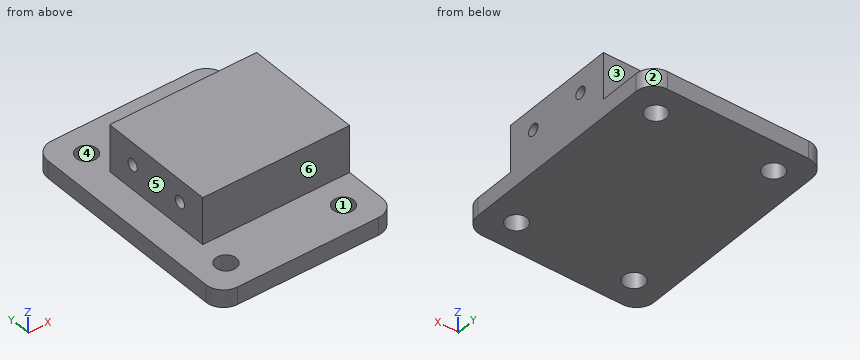
from build123d import *

# Parameters (mm, degrees)
SKETCH_1_W              = 30
SKETCH_1_H              = 40
EXTRUDE_1_DEPTH         = 1.5
SKETCH_2_W              = 25
SKETCH_2_H              = 20
EXTRUDE_2_DEPTH         = 8
HOLE_WIZARD_2_0_2_3_D   = 2
HOLE_WIZARD_3_5_3_5_1_D = 3.5
FILLET_1_R              = 3


with BuildPart() as part:
    # 草圖1 → 填料-伸長1 (new, symmetric)
    with BuildSketch(Plane.XY):
        Rectangle(SKETCH_1_W, SKETCH_1_H)
    extrude(amount=EXTRUDE_1_DEPTH, both=True)

    # 草圖2 → 填料-伸長2 (add)
    with BuildSketch(Plane.XY.offset(1.5)):
        with Locations((2.5, 0)):
            Rectangle(SKETCH_2_W, SKETCH_2_H)
    extrude(amount=EXTRUDE_2_DEPTH)

    # Ø2.0 (2) 直徑孔3 (through all)
    with Locations(Plane.ZY.offset(10)):
        with Locations((5.69, 5.08), (5.69, -5.08)):
            Hole(HOLE_WIZARD_2_0_2_3_D / 2)

    # Ø3.5 (3.5) 直徑孔1 (through all)
    with Locations(Plane.XY.offset(1.5)):
        with Locations((10, 15), (-10, -15), (-10, 15), (10, -15)):
            Hole(HOLE_WIZARD_3_5_3_5_1_D / 2)

    # 圓角1
    fillet_1_edges = [part.edges().sort_by_distance(p)[0] for p in [
        (15, -20, 0),
        (-15, -20, 0),
        (-15, 20, 0),
        (15, 20, 0),
    ]]
    fillet(fillet_1_edges, radius=FILLET_1_R)


solid = part.part
Can you work these out from the model? Positions are in its coordinate system, mm. Face numbers are marked on the shaded views. A direction names the side the tool comes from. Give positions to 0.01 mm unless a question says otherwise; leave off trailing zeros. Loops run counter-clockwise (first coordinate to the right, second up) from the corner with the lowest first, then second, coordinate; pieces in that order, holes last. Notation, with made-up numbers: M -15,31 L 37,31 A21 ccw 37,67 Z; hole C 62.5,78 d8. An arc over 180 degrees is marked long. One line per item, written item: value. Start each with the question number.
1) I'm going to push flat-ended pins straight in: pin 1 (4 mm diameter, centred on x = -3.5, z = 7.5, fed in from -Y); pin 2 (3 mm diameter, centred on y = 10.5, z = 6.5, fed in from -X); pin 3 (4 mm diameter, centred on x = 10, y = -15, fed in from +Z). Where does each tip first touch, or does it pass through?
2) If we section it at A-A, the plane x = -6.5: Write out the boundary of the cut face in (y, z).
3) If we section it at D-D, the plane y = 5.08: Write out the boundary of the cut face in (x, z), and give its area (3 significant figures).
4) On a 3-axis mill with a long thin cutter (end or side, diameter ignored), from which of +Z, -Z, +X, -X, +Y, -Y can I reach the whole of each face in a straight line? I mean the marked faces 4, 5 and 6. Say none if no direction works.
5) If I drill on line 1 (Y direction, x = 10, z = -0.05); line 2 (Y direction, x = 5.75, z = 6); line 3 (Y direction, x = -5.5, z = 8), over which ranges is the centre line in solid material (lowest first)? Write a range as [from, to].
6) If we section it at B-B, the plane z = 0: Write out the boundary of the cut face in (x, y), and give its area (3 significant figures).
7) If we section it at C-C, the plane x = 10: Write out the boundary of the cut face in (y, z), and give its area (3 significant figures).
8) Thinking about a two-plate mould opening in X: for the marked faces 1, 2 and 3, which applies, +X half, -X half, draft (parallel to the pull), parting line (faces both ways), or undercut?
Completed:
1. pin 1: stops at y = -10
1. pin 2: stops at x = -10
1. pin 3: stops at z = 1.5
2. outline: M -20,-1.5 L 20,-1.5 L 20,1.5 L 10,1.5 L 10,9.5 L -10,9.5 L -10,1.5 L -20,1.5 Z; hole C -5.08,5.69 d2; hole C 5.08,5.69 d2
3. outline: M -15,-1.5 L 15,-1.5 L 15,4.69 L -10,4.69 L -10,1.5 L -15,1.5 Z; M -10,6.69 L 15,6.69 L 15,9.5 L -10,9.5 Z
3. area: 240 mm^2
4. face 4: +Z, -Z
4. face 5: +Z, -X, +Y, -Y
4. face 6: +Z, +X, -X, -Y
5. line 1: y = [-20, -16.75], [-13.25, 13.25], [16.75, 20]
5. line 2: y = [-10, -6.03], [-4.13, 4.13], [6.03, 10]
5. line 3: y = [-10, 10]
6. outline: M -15,-17 A3 ccw -12,-20 L 12,-20 A3 ccw 15,-17 L 15,17 A3 ccw 12,20 L -12,20 A3 ccw -15,17 Z; hole C -10,-15 d3.5; hole C -10,15 d3.5; hole C 10,-15 d3.5; hole C 10,15 d3.5
6. area: 1,150 mm^2
7. outline: M -20,-1.5 L -16.75,-1.5 L -16.75,1.5 L -20,1.5 Z; M -13.25,-1.5 L 13.25,-1.5 L 13.25,1.5 L 10,1.5 L 10,9.5 L -10,9.5 L -10,1.5 L -13.25,1.5 Z; M 16.75,-1.5 L 20,-1.5 L 20,1.5 L 16.75,1.5 Z; hole C -5.08,5.69 d2; hole C 5.08,5.69 d2
7. area: 253 mm^2
8. face 1: undercut
8. face 2: +X half
8. face 3: draft
